The model under review builds one solid part; all positions refer to its coordinate system, in mm. Coordinates: 2 decimals unless noted, no trailing zeros. Write each loop counter-clockwise with the first axis right and the second up, starting at its lowest first coordinate (ties: lowest second). Pieces come first, ordered by that corner, then holes.
1) Add section A-A, the plane x = -18.5. State the section outline as (y, z) points, then the cut area to 3 significant figures.
2) For line 1 (Z direction, x = -18.5, y = 0.3); line 2 (X direction, y = 4.65, z = -27) (3 decimals); line 3 (Z direction, x = 12, y = 4.4), list the stretches that pass through material, from the lowest coordinate up.
3) Add section C-C, the plane z = -27. State the section outline as (x, y) points (3 decimals).
4) Add section B-B, the plane z = -15. State the section outline as (x, y) points.
5) Add section D-D, the plane x = 21. State the section outline as (y, z) points, then the cut area to 3 significant figures.
6) For P1, Ø1.8, axis at x = 16, y = 3.5, coming from the -Z side; P2, Ø1.8, axis at y = 3, z = 28.5, coming from the +X side; P3, Ø1.8, axis at y = 3.5, z = 27.5, coming from the +X side, all flat-tipped, find the tip position at first contact; note any pin that passes through.
from build123d import *

# Parameters (mm, degrees)
EXTRUDE_1_DEPTH      = 6
SKETCH_2_R           = 2.55
SKETCH_2_R_2         = 1.6
CUT_EXTRUDE_1_DEPTH  = 7
CUT_EXTRUDE_2_DEPTH  = 7
EXTRUDE_2_DEPTH      = 6
SKETCH_31_R          = 2.1
SKETCH_31_W          = 7
SKETCH_31_H          = 6
CUT_EXTRUDE_11_DEPTH = 7
EXTRUDE_21_DEPTH     = 6
SKETCH_33_R          = 2.1
SKETCH_33_W          = 7
SKETCH_33_H          = 6
CUT_EXTRUDE_13_DEPTH = 7


with BuildPart() as part:
    # Эскиз1 → Бобышка-Вытянуть1 (new body)
    with BuildSketch(Plane(origin=(0, 0, 0), x_dir=(1, 0, 0), z_dir=(0, 1, 0))):
        with BuildLine():
            Line((-27, -30), (27, -30))
            ThreePointArc((27, -30), (32.656854249, -27.656854249), (35, -22))
            Line((35, -22), (35, 22))
            ThreePointArc((35, 22), (32.656854249, 27.656854249), (27, 30))
            Line((27, 30), (-27, 30))
            ThreePointArc((-27, 30), (-32.656854249, 27.656854249), (-35, 22))
            Line((-35, 22), (-35, -22))
            ThreePointArc((-35, -22), (-32.656854249, -27.656854249), (-27, -30))
        make_face()
    extrude(amount=EXTRUDE_1_DEPTH)

    # Эскиз2 → Вырез-Вытянуть1 (cut, through all)
    with BuildSketch(Plane.XZ):
        with Locations((-25, -15)):
            Circle(SKETCH_2_R)
        with Locations((-25, 15)):
            Circle(SKETCH_2_R)
        with Locations((12, 19.966651117)):
            Circle(SKETCH_2_R_2)
        with Locations((12, -19.966651117)):
            Circle(SKETCH_2_R_2)
        with BuildLine():
            Line((28, -17.55), (26, -17.55))
            ThreePointArc((26, -17.55), (23.45, -15), (26, -12.45))
            Line((26, -12.45), (28, -12.45))
            ThreePointArc((28, -12.45), (30.55, -15), (28, -17.55))
        make_face()
        with BuildLine():
            Line((28, 17.55), (26, 17.55))
            ThreePointArc((26, 17.55), (23.45, 15), (26, 12.45))
            Line((26, 12.45), (28, 12.45))
            ThreePointArc((28, 12.45), (30.55, 15), (28, 17.55))
        make_face()
    extrude(amount=-CUT_EXTRUDE_1_DEPTH, mode=Mode.SUBTRACT)

    # Эскиз3 → Вырез-Вытянуть2 (cut, through all)
    with BuildSketch(Plane.XZ):
        with BuildLine():
            Line((-35, -2), (-35, 2))
            ThreePointArc((-35, 2), (-34.414213562, 0.585786438), (-33, 0))
            ThreePointArc((-33, 0), (-34.414213562, -0.585786438), (-35, -2))
        make_face()
    extrude(amount=-CUT_EXTRUDE_2_DEPTH, mode=Mode.SUBTRACT)

    # Эскиз21 → Бобышка-Вытянуть2 (add)
    with BuildSketch(Plane(origin=(-9.322772353, 6, 20), x_dir=(-1, 0, 0), z_dir=(0, -1, 0))):
        with BuildLine():
            Line((13, 53), (-13, 53))
            ThreePointArc((-13, 53), (-14.118033989, 52.736067977), (-15, 52))
            Line((-15, 52), (-16.2, 50.4))
            ThreePointArc((-16.2, 50.4), (-16.552786405, 50.105572809), (-17, 50))
            Line((-17, 50), (17, 50))
            ThreePointArc((17, 50), (16.552786405, 50.105572809), (16.2, 50.4))
            Line((16.2, 50.4), (15, 52))
            ThreePointArc((15, 52), (14.118033989, 52.736067977), (13, 53))
        make_face()
    extrude(amount=EXTRUDE_2_DEPTH)

    # Эскиз31 → Вырез-Вытянуть11 (cut, through all)
    with BuildSketch(Plane(origin=(-9.322772353, 0, 20), x_dir=(-1, 0, 0), z_dir=(0, -1, 0))):
        with Locations((0, 47)):
            Circle(SKETCH_31_R)
        with Locations((9.531849908, 47)):
            Rectangle(SKETCH_31_W, SKETCH_31_H)
        with Locations((-9.531849908, 47)):
            Rectangle(SKETCH_31_W, SKETCH_31_H)
    extrude(amount=-CUT_EXTRUDE_11_DEPTH, mode=Mode.SUBTRACT)

    # Эскиз22 → Бобышка-Вытянуть21 (add)
    with BuildSketch(Plane(origin=(-9.322772353, 6, -20), x_dir=(1, 0, 0), z_dir=(0, -1, 0))):
        with BuildLine():
            Line((13, 53), (-13, 53))
            ThreePointArc((-13, 53), (-14.118033989, 52.736067977), (-15, 52))
            Line((-15, 52), (-16.2, 50.4))
            ThreePointArc((-16.2, 50.4), (-16.552786405, 50.105572809), (-17, 50))
            Line((-17, 50), (17, 50))
            ThreePointArc((17, 50), (16.552786405, 50.105572809), (16.2, 50.4))
            Line((16.2, 50.4), (15, 52))
            ThreePointArc((15, 52), (14.118033989, 52.736067977), (13, 53))
        make_face()
    extrude(amount=EXTRUDE_21_DEPTH)

    # Эскиз33 → Вырез-Вытянуть13 (cut, through all)
    with BuildSketch(Plane(origin=(-9.322772353, 0, -20), x_dir=(1, 0, 0), z_dir=(0, -1, 0))):
        with Locations((0, 47)):
            Circle(SKETCH_33_R)
        with Locations((9.531849908, 47)):
            Rectangle(SKETCH_33_W, SKETCH_33_H)
        with Locations((-9.531849908, 47)):
            Rectangle(SKETCH_33_W, SKETCH_33_H)
    extrude(amount=-CUT_EXTRUDE_13_DEPTH, mode=Mode.SUBTRACT)


solid = part.part
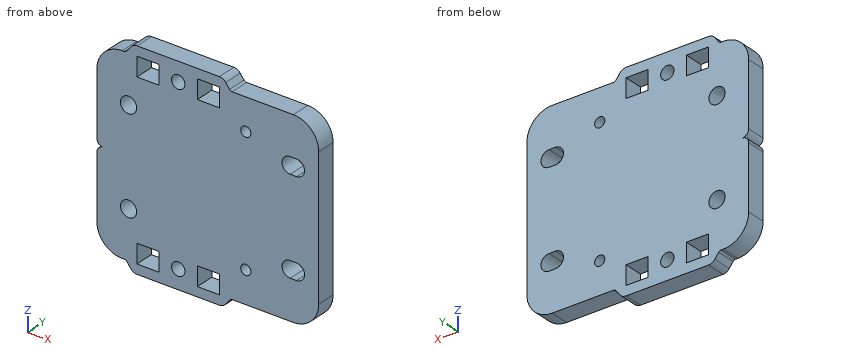
Geometry results:
1. outline: (0, -33) - (6, -33) - (6, -30) - (0, -30) - close; (0, -24) - (6, -24) - (6, 24) - (0, 24) - close; (0, 30) - (6, 30) - (6, 33) - (0, 33) - close
1. area: 324 mm2
2. line 1: z = -33 to -30, -24 to 24, 30 to 33
2. line 2: x = -33.245 to -22.355, -15.355 to -11.423, -7.223 to -3.291, 3.709 to 33.245
2. line 3: z = -30 to -21.57, -18.37 to 18.37, 21.57 to 30
3. outline: (-33.245, 0) - (-22.355, 0) - (-22.355, 6) - (-33.245, 6) - close; (-15.355, 0) - (-11.423, 0) - (-11.423, 6) - (-15.355, 6) - close; (-7.223, 0) - (-3.291, 0) - (-3.291, 6) - (-7.223, 6) - close; (3.709, 0) - (33.245, 0) - (33.245, 6) - (3.709, 6) - close
4. outline: (-35, 0) - (-27.55, 0) - (-27.55, 6) - (-35, 6) - close; (-22.45, 0) - (23.45, 0) - (23.45, 6) - (-22.45, 6) - close; (30.55, 0) - (35, 0) - (35, 6) - (30.55, 6) - close
5. outline: (0, -30) - (6, -30) - (6, 30) - (0, 30) - close
5. area: 360 mm2
6. P1: stops at z = -30
6. P2: stops at x = 32.71
6. P3: stops at x = 33.55
